from build123d import *

# Parameters (mm, degrees)
SKETCH1_W                  = 310
SKETCH1_H                  = 130
BOSS_EXTRUDE1_DEPTH        = 3
CUT_EXTRUDE2_DEPTH         = 4
FILLET1_R                  = 4
F_5_3_5_3_DIAMETER_HOLE1_D = 5.3
SKETCH6_R                  = 5
SKETCH6_W                  = 12
SKETCH6_H                  = 10
CUT_EXTRUDE1_DEPTH         = 4
FILLET2_R                  = 2
CUT_EXTRUDE3_DEPTH         = 4


with BuildPart() as part:
    # Sketch1 → Boss-Extrude1 (new body)
    with BuildSketch(Plane(origin=(0, 0, 0), x_dir=(1, 0, 0), z_dir=(0, 1, 0))):
        Rectangle(SKETCH1_W, SKETCH1_H)
    extrude(amount=BOSS_EXTRUDE1_DEPTH)

    # Sketch7 → Cut-Extrude2 (cut, through all)
    with BuildSketch(Plane(origin=(0, 3, 0), x_dir=(1, 0, 0), z_dir=(0, 1, 0))):
        Polygon((-155, 65), (-155, 45), (-135, 65), align=None)
        Polygon((135, 65), (155, 65), (155, 45), align=None)
        Polygon((155, -65), (155, -45), (135, -65), align=None)
        Polygon((-135, -65), (-155, -65), (-155, -45), align=None)
    extrude(amount=-CUT_EXTRUDE2_DEPTH, mode=Mode.SUBTRACT)

    # Fillet1
    fillet1_edges = [part.edges().sort_by_distance(p)[0] for p in [
        (-155, 1.5, 45),
        (-135, 1.5, 65),
        (135, 1.5, 65),
        (155, 1.5, 45),
        (155, 1.5, -45),
        (135, 1.5, -65),
        (-135, 1.5, -65),
        (-155, 1.5, -45),
    ]]
    fillet(fillet1_edges, radius=FILLET1_R)

    # Ø5.3 (5.3) Diameter Hole1 (through all)
    with Locations(Plane(origin=(0, 3, 0), x_dir=(1, 0, 0), z_dir=(0, 1, 0))):
        with Locations((125, 55), (-125, -55), (-125, 55), (125, -55)):
            Hole(F_5_3_5_3_DIAMETER_HOLE1_D / 2)

    # Sketch6 → Cut-Extrude1 (cut, through all)
    with BuildSketch(Plane(origin=(0, 3, 0), x_dir=(1, 0, 0), z_dir=(0, 1, 0))):
        with Locations((115, -35)):
            Circle(SKETCH6_R)
        with Locations((95, -35)):
            Rectangle(SKETCH6_W, SKETCH6_H)
    extrude(amount=-CUT_EXTRUDE1_DEPTH, mode=Mode.SUBTRACT)

    # Fillet2
    fillet2_edges = [part.edges().sort_by_distance(p)[0] for p in [
        (101, 1.5, 30),
        (101, 1.5, 40),
        (89, 1.5, 40),
        (89, 1.5, 30),
    ]]
    fillet(fillet2_edges, radius=FILLET2_R)

    # Sketch8 → Cut-Extrude3 (cut, through all)
    with BuildSketch(Plane(origin=(0, 3, 0), x_dir=(1, 0, 0), z_dir=(0, 1, 0))):
        with BuildLine():
            Line((-127.65, 53.5), (-127.65, 56.5))
            ThreePointArc((-127.65, 56.5), (-125, 59.15), (-122.35, 56.5))
            Line((-122.35, 56.5), (-122.35, 53.5))
            ThreePointArc((-122.35, 53.5), (-125, 50.85), (-127.65, 53.5))
        make_face()
        with BuildLine():
            Line((122.35, 53.5), (122.35, 56.5))
            ThreePointArc((122.35, 56.5), (125, 59.15), (127.65, 56.5))
            Line((127.65, 56.5), (127.65, 53.5))
            ThreePointArc((127.65, 53.5), (125, 50.85), (122.35, 53.5))
        make_face()
    extrude(amount=-CUT_EXTRUDE3_DEPTH, mode=Mode.SUBTRACT)


solid = part.part
Check sheet for the modelled part. Datum: model origin and axes. Units: mm. Give positions to 0.01 mm unless a question says otherwise; leave off trailing zeros. Write each loop counter-clockwise with the first axis right and the second up, starting at its lowest first coordinate (ties: lowest second). Pieces come first, ordered by that corner, then holes. Notation, with made-up numbers: (-20.5, 20.25) -> (-5.5, 20.25) arc R18 cw to (-5.5, 30.25) -> close; hole circle Ø9 at (-31.5, 44). An arc over 180 degrees is marked (long way). Use one line per item in the form item = value. Start each with the question number.
1. Section check B-B (x = 115). Record the cut outline in (y, z).
2. Section check A-A (z = 35). Record the cut outline in (x, y).
3. Section check C-C (y = 0.85). Count the separate pieces of the cut face and the enclosed holes in it, and give its area (3 significant figures).
4. Go/stop test with flat-tipped pins: P1, Ø0.9, axis at y = 2, z = -55, coming from the -X side; P2, Ø1.5, axis at y = 1.5, z = -55, coming from the -X side. Record where each tip stops, or that it passes through.
5. Thickness scan on line 1 along Z through (x, y) = (125, 2.1); line 2 along X through (y, z) = (0.9, 35); line 3 along X through (y, z) = (1.5, 55). Record the ranges inside material, lowest first. Write a range as from..to.
6. Mould release check, pull along X, two halves, no side actions. Record for faces 1 (the flat face through (145, 2, -55)), 2 (the cylindrical face through (122.472, 1.479, 54.204)), 3 (the flat face through (-2, 0, -1)): pulls with the +X half, pulls with the -X half, needs draft (parallel to the pull), parting line crosses it, or undercut.
Conclusion:
q1.outline = (0, -65) -> (3, -65) -> (3, 30) -> (0, 30) -> close; (0, 40) -> (3, 40) -> (3, 65) -> (0, 65) -> close
q2.outline = (-155, 0) -> (89, 0) -> (89, 3) -> (-155, 3) -> close; (101, 0) -> (110, 0) -> (110, 3) -> (101, 3) -> close; (120, 0) -> (155, 0) -> (155, 3) -> (120, 3) -> close
q3.separate_pieces = 1
q3.enclosed_holes = 6
q3.area = 39,200 mm²
q4.P1 = -145.45
q4.P2 = -145.75
q5.line_1 = -65..-59.15, -50.85..52.35, 57.65..65
q5.line_2 = -155..89, 101..110, 120..155
q5.line_3 = -145..-127.65, -122.35..122.35, 127.65..145
q6.face_1 = pulls with the +X half
q6.face_2 = undercut
q6.face_3 = needs draft
